Geometry check sheet. Reference: the model listing, model coordinates, mm. Face numbers are marked on the shaded views. A direction names the side the tool comes from. Coordinates: 2 decimals unless noted, no trailing zeros. Order: outer loops, then holes, each group sorted by start corner. A loop starts at its lowest first (then second) coordinate and runs counter-clockwise, first axis right, second up. Notation, with made-up numbers: M 56.5,29.25 L 69.5,29.25 A23 cw 69.5,53.25 Z; hole C 30.25,-8.75 d5. An arc over 180 degrees is marked long. One line per item, written item: value. Start each with the question number.
1) Sectioned sample at A-A, the plane y = 0.4. Enter the section's corners in (x, z), then the cut area to 3 significant figures.
2) Sectioned sample at D-D, the plane x = 3.5. Enter the section's corners in (y, z), then the cut area to 3 significant figures.
3) Sectioned sample at C-C, the plane y = 2.05. Enter the section's corners in (x, z).
4) Sectioned sample at B-B, the plane x = 0. Enter the section's corners in (y, z), then the cut area to 3 significant figures.
5) Go/stop test with a flat-tipped pin: P1, Ø2, axis at x = 4, z = 1.5, coming from the +Y side. Record where the tip stops, or that it passes through.
6) Thickness scan on L1, parallel to X at y = 1, z = -4.5; L2, parallel to Y at x = -2.25, z = -4.5; L3, parallel to Z at x = -5.5, y = 0.7. Record the ranges inside material, lowest first. Write a range as from..to.
7) Access from +Z, -Z, +X, -X, +Y, -Y to the whole of each face (thin tool, end or side, straight path). Record for the marked faces 1 and 2.
```python
from build123d import *

# Parameters (mm, degrees)
SALIENTE_EXTRUIR1_DEPTH = 1.5
CROQUIS3_R              = 2.5
SALIENTE_EXTRUIR2_DEPTH = 1
REDONDEO2_R             = 0.5
REDONDEO3_R             = 0.2


with BuildPart() as part:
    # Croquis2 → Saliente-Extruir1 (new body)
    with BuildSketch(Plane(origin=(0, 0, 0), x_dir=(1, 0, 0), z_dir=(0, 1, 0))):
        with BuildLine():
            Line((-5.014556606, 6.035834257), (4.79615183, 6.035834257))
            ThreePointArc((4.79615183, 6.035834257), (5.152675046, 5.725750413), (5.489639121, 5.394516348))
            Line((5.489639121, 5.394516348), (4.737625192, 4.763501737))
            Line((4.737625192, 4.763501737), (5.388283977, 3.988076792))
            Line((5.388283977, 3.988076792), (6.140297907, 4.619091403))
            ThreePointArc((6.140297907, 4.619091403), (7.640797612, 0.035834257), (6.140297907, -4.547422889))
            Line((6.140297907, -4.547422889), (5.388283977, -3.916408278))
            Line((5.388283977, -3.916408278), (4.737625192, -4.691833224))
            Line((4.737625192, -4.691833224), (5.489639121, -5.322847835))
            ThreePointArc((5.489639121, -5.322847835), (5.152675046, -5.6540819), (4.79615183, -5.964165743))
            Line((4.79615183, -5.964165743), (-5.014556606, -5.964165743))
            ThreePointArc((-5.014556606, -5.964165743), (-5.371079822, -5.6540819), (-5.708043897, -5.322847835))
            Line((-5.708043897, -5.322847835), (-4.956029967, -4.691833224))
            Line((-4.956029967, -4.691833224), (-5.606688753, -3.916408278))
            Line((-5.606688753, -3.916408278), (-6.358702683, -4.547422889))
            ThreePointArc((-6.358702683, -4.547422889), (-7.859202388, 0.035834257), (-6.358702683, 4.619091403))
            Line((-6.358702683, 4.619091403), (-5.606688753, 3.988076792))
            Line((-5.606688753, 3.988076792), (-4.956029967, 4.763501737))
            Line((-4.956029967, 4.763501737), (-5.708043897, 5.394516348))
            ThreePointArc((-5.708043897, 5.394516348), (-5.371079822, 5.725750413), (-5.014556606, 6.035834257))
        make_face()
    extrude(amount=SALIENTE_EXTRUIR1_DEPTH)

    # Croquis3 → Saliente-Extruir2 (add)
    with BuildSketch(Plane(origin=(0, 1.5, 0), x_dir=(1, 0, 0), z_dir=(0, 1, 0))):
        with Locations(Location((0, 0, 0), (0, 0, 270))):
            Circle(CROQUIS3_R)
    extrude(amount=SALIENTE_EXTRUIR2_DEPTH)

    # Redondeo2
    redondeo2_edges = [part.edges().sort_by_distance(p)[0] for p in [
        (-7.859202388, 1.5, -0.035834257),
        (-5.371079822, 1.5, 5.6540819),
        (-0.109202388, 1.5, 5.964165743),
        (5.152675046, 1.5, 5.6540819),
        (-5.371079822, 1.5, -5.725750413),
        (7.640797612, 1.5, -0.035834257),
        (5.152675046, 1.5, -5.725750413),
        (-0.109202388, 1.5, -6.035834257),
    ]]
    fillet(redondeo2_edges, radius=REDONDEO2_R)

    # Redondeo3
    redondeo3_edges = [part.edges().sort_by_distance(p)[0] for p in [
        (0, 2.5, -2.5),
    ]]
    fillet(redondeo3_edges, radius=REDONDEO3_R)


solid = part.part
```
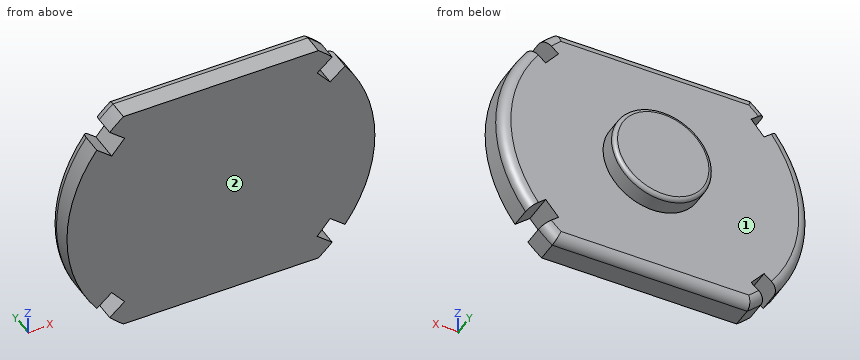
Final values:
1. outline: M -6.36,-4.62 L -5.61,-3.99 L -4.96,-4.76 L -5.71,-5.39 A7.75 ccw -5.01,-6.04 L 4.8,-6.04 A7.75 ccw 5.49,-5.39 L 4.74,-4.76 L 5.39,-3.99 L 6.14,-4.62 A7.75 ccw 6.14,4.55 L 5.39,3.92 L 4.74,4.69 L 5.49,5.32 A7.75 ccw 4.8,5.96 L -5.01,5.96 A7.75 ccw -5.71,5.32 L -4.96,4.69 L -5.61,3.92 L -6.36,4.55 A7.75 ccw Z
1. area: 161 mm^2
2. outline: M 0,-6.04 L 1,-6.04 A0.5 ccw 1.5,-5.54 L 1.5,5.46 A0.5 ccw 1,5.96 L 0,5.96 Z
2. area: 17.9 mm^2
3. outline: C 0,0 d5
4. outline: M 0,-6.04 L 1,-6.04 A0.5 ccw 1.5,-5.54 L 1.5,-2.5 L 2.3,-2.5 A0.2 ccw 2.5,-2.3 L 2.5,2.3 A0.2 ccw 2.3,2.5 L 1.5,2.5 L 1.5,5.46 A0.5 ccw 1,5.96 L 0,5.96 Z
4. area: 22.9 mm^2
5. P1: stops at y = 1.5
6. L1: x = -6.44..-6.22, -5.18..4.96, 6..6.23
6. L2: y = 0..1.5
6. L3: z = -5.6..-5.22, -4.12..4.04, 5.15..5.53
7. face 1: +Y
7. face 2: +Z, -Z, +X, -X, -Y
